For this review, take the finished solid that the model builds, in its own axes (mm). A direction names the side the tool comes from. Coordinates: 2 decimals unless noted, no trailing zeros. Write each loop counter-clockwise with the first axis right and the second up, starting at its lowest first coordinate (ties: lowest second). Pieces come first, ordered by that corner, then holes. Notation, with made-up numbers: (-4.75, 62) - (2.25, 62) arc R33 ccw to (2.25, 96) - close; hole circle Ø7 at (-3, 67). An arc over 180 degrees is marked (long way). Write each question's results on one line, items separated by ' | '.
from build123d import *

# Parameters (mm, degrees)
SKETCH_1_R           = 37.5
EXTRUDE_1_DEPTH      = 10
EXTRUDE_2_DEPTH      = 10
EXTRUDE_2_DEPTH_BACK = 10
FILLET_1_R           = 5
FILLET_2_R           = 10


with BuildPart() as part:
    # 草图1 → 凸台-拉伸1 (new body)
    with BuildSketch(Plane(origin=(0, 0, 0), x_dir=(1, 0, 0), z_dir=(0, 1, 0))):
        with Locations(Location((0, 0, 0), (0, 0, 270))):
            Circle(SKETCH_1_R)
    extrude(amount=EXTRUDE_1_DEPTH)

    # 草图2 → 凸台-拉伸2 (add, two sides: drawn at the far end of the back side and taken through both)
    with BuildSketch(Plane.XY.offset(-EXTRUDE_2_DEPTH_BACK)):
        with BuildLine():
            Line((15, 0), (15, 20))
            Line((15, 20), (40, 34.43375673))
            Line((40, 34.43375673), (40, 102.679491924))
            Line((40, 102.679491924), (33.660254038, 113.660254038))
            Line((33.660254038, 113.660254038), (25, 108.660254038))
            Line((25, 108.660254038), (30, 100))
            Line((30, 100), (30, 40))
            ThreePointArc((30, 40), (0, 27.573593129), (-30, 40))
            Line((-30, 40), (-30, 100))
            Line((-30, 100), (-25, 108.660254038))
            Line((-25, 108.660254038), (-33.660254038, 113.660254038))
            Line((-33.660254038, 113.660254038), (-40, 102.679491924))
            Line((-40, 102.679491924), (-40, 34.43375673))
            Line((-40, 34.43375673), (-15, 20))
            Line((-15, 20), (-15, 0))
            Line((-15, 0), (15, 0))
        make_face()
    extrude(amount=EXTRUDE_2_DEPTH + EXTRUDE_2_DEPTH_BACK)

    # 圆角1
    fillet_1_edges = [part.edges().sort_by_distance(p)[0] for p in [
        (33.660254038, 113.660254038, 0),
        (25, 108.660254038, 0),
        (-25, 108.660254038, 0),
        (-33.660254038, 113.660254038, 0),
    ]]
    fillet(fillet_1_edges, radius=FILLET_1_R - 0.0001)  # a hair under: the kernel refuses the full size

    # 圆角2
    fillet_2_edges = [part.edges().sort_by_distance(p)[0] for p in [
        (-40, 34.43375673, 0),
        (-40, 102.679491924, 0),
        (40, 102.679491924, 0),
        (40, 34.43375673, 0),
    ]]
    fillet(fillet_2_edges, radius=FILLET_2_R)


solid = part.part
Q1. Take a section at A-A on x = 0. State the section outline as (y, z) points, plus the area to 3 significant figures.
Results found:
outline: (0, -37.5) - (10, -37.5) - (10, -10) - (27.57, -10) - (27.57, 10) - (10, 10) - (10, 37.5) - (0, 37.5) - close | area: 1,100 mm2
Q2. For faces 1 (the face through (-38.697, 35.271, 0.14)), 2 (the face through (0, 27, -10)), 3 (the face through (38.62, 35.14, 0.14)), 4 (the face through (28.73, 102.2, -0.14)), list the 3-axis set-ups (+Z, -Z, +X, -X, +Y, -Y) from which the entire face can be reached by the end or side of a thin tool; tool diameter is ignored.
Results found:
face 1: +Z, -Z, -X | face 2: -Z, +X, -X, +Y | face 3: +Z, -Z, +X | face 4: +Z, -Z
Q3. Take a section at D-D on x = -8. State the section outline as (y, z) points, plus the area to 3 significant figures.
Results found:
outline: (0, -36.64) - (10, -36.64) - (10, -10) - (28.33, -10) - (28.33, 10) - (10, 10) - (10, 36.64) - (0, 36.64) - close | area: 1,100 mm2
Q4. Take a section at C-C on y = 13. State the section outline as (x, z) points.
Results found:
outline: (-15, -10) - (15, -10) - (15, 10) - (-15, 10) - close
Q5. For pin 1 (2 mm diameter, centred on y = 21.5, z = -10.5, fed in from -X); pin 2 (3 mm diameter, centred on y = 16, z = -3.5, fed in from +X); pin 3 (10 mm diameter, centred on x = -16, z = 20.5, fed in from +Y), all flat-tipped, find the tip position at first contact; note any pin that passes through.
Results found:
pin 1: x = -19.1 | pin 2: x = 15 | pin 3: y = 10
Q6. Mouldability with a two-part tool opening along Y and no side actions: class faces 5 (the face through (-1, 0, -1)), 6 (the face through (26.987, 108.071, 0.14)), 7 (the face through (-40, 71, 0)) as pulls with the +Y half, pulls with the -Y half, needs draft (parallel to the pull), parting line crosses it, or undercut.
Results found:
face 5: pulls with the -Y half | face 6: undercut | face 7: needs draft
Q7. Wall thickness on line 1 along X through (y, z) = (45, 8); line 2 along Z through (x, y) = (-34.5, 85.5); line 3 along Y through (x, z) = (19, 30): over which ranges is each line inside the solid? List them lowest first. Write a range as from..to.
Results found:
line 1: -40..-30, 30..40 | line 2: -10..10 | line 3: 0..10
